Build history of the part. All positions in model axes, mm. A direction names the side the tool comes from. Round coordinates to 2 decimals unless told otherwise and drop trailing zeros. Write each loop counter-clockwise with the first axis right and the second up, starting at its lowest first coordinate (ties: lowest second). Pieces come first, ordered by that corner, then holes. Notation, with made-up numbers: M 61,2 L 69,2 A23 ccw 69,24 Z; hole C 17.25,83.5 d9. An arc over 180 degrees is marked long. Write item = value, one per line.
from build123d import *

# Parameters (mm, degrees)
SKETCH1_W           = 304.8
SKETCH1_H           = 381
BOSS_EXTRUDE1_DEPTH = 152.4
SKETCH2_R           = 38.1
CUT_EXTRUDE1_DEPTH  = 50.8
SKETCH5_W           = 152.4
SKETCH5_H           = 101.6
BOSS_EXTRUDE3_DEPTH = 127
SKETCH6_R           = 25.4
CUT_EXTRUDE4_DEPTH  = 50.8
FILLET4_R           = 25.4
FILLET5_R           = 25.4
SKETCH3_R           = 38.1
BOSS_EXTRUDE4_DEPTH = 44.45
SKETCH8_W           = 122.871403684
SKETCH8_H           = 31.75
CUT_EXTRUDE5_DEPTH  = 63.5
SKETCH9_R           = 12.7
BOSS_EXTRUDE5_DEPTH = 32.766


with BuildPart() as part:
    # Sketch1 → Boss-Extrude1 (new body)
    with BuildSketch(Plane.XY):
        Rectangle(SKETCH1_W, SKETCH1_H)
    extrude(amount=BOSS_EXTRUDE1_DEPTH)

    # Sketch2 → Cut-Extrude1 (cut)
    with BuildSketch(Plane(origin=(0, 190.5, 0), x_dir=(1, 0, 0), z_dir=(0, 1, 0))):
        with Locations(Location((0, -76.2, 0), (0, 0, 270))):
            Circle(SKETCH2_R)
    extrude(amount=-CUT_EXTRUDE1_DEPTH, mode=Mode.SUBTRACT)

    # Sketch5 → Boss-Extrude3 (add)
    with BuildSketch(Plane(origin=(152.4, 0, 0), x_dir=(0, 0, -1), z_dir=(1, 0, 0))):
        with Locations((-76.2, 139.7)):
            Rectangle(SKETCH5_W, SKETCH5_H)
    boss_extrude3 = extrude(amount=BOSS_EXTRUDE3_DEPTH)

    # Mirror1: Boss-Extrude3 across plane
    add(boss_extrude3.mirror(Plane(origin=(0, 0, 0), x_dir=(0, 0, 1), z_dir=(1, 0, 0))))

    # Sketch6 → Cut-Extrude4 (cut)
    with BuildSketch(Plane.XZ.offset(-88.9)):
        with Locations(Location((228.6, 76.2, 0), (0, 0, 270))):
            Circle(SKETCH6_R)
    cut_extrude4 = extrude(amount=-CUT_EXTRUDE4_DEPTH, mode=Mode.SUBTRACT)

    # Fillet4
    fillet4_edges = [part.edges().sort_by_distance(p)[0] for p in [
        (279.4, 190.5, 76.2),
        (-279.4, 190.5, 76.2),
    ]]
    fillet(fillet4_edges, radius=FILLET4_R)

    # Fillet5
    fillet5_edges = [part.edges().sort_by_distance(p)[0] for p in [
        (-152.4, -190.5, 76.2),
        (152.4, -190.5, 76.2),
    ]]
    fillet(fillet5_edges, radius=FILLET5_R)

    # Mirror2: Cut-Extrude4 across plane
    add(cut_extrude4.mirror(Plane(origin=(0, 0, 0), x_dir=(0, 0, 1), z_dir=(1, 0, 0))), mode=Mode.SUBTRACT)

    # Sketch3 → Boss-Extrude4 (add)
    with BuildSketch(Plane.XZ.offset(190.5)):
        with Locations(Location((-101.6, 76.2, 0), (0, 0, 131.810314896))):
            Circle(SKETCH3_R)
        with Locations(Location((101.6, 76.2, 0), (0, 0, 48.189685104))):
            Circle(SKETCH3_R)
    extrude(amount=BOSS_EXTRUDE4_DEPTH)

    # Sketch8 → Cut-Extrude5 (cut)
    with BuildSketch(Plane.XZ.offset(234.95)):
        with Locations((101.6, 76.2)):
            Rectangle(SKETCH8_W, SKETCH8_H)
    cut_extrude5 = extrude(amount=-CUT_EXTRUDE5_DEPTH, mode=Mode.SUBTRACT)

    # Mirror3: Cut-Extrude5 across plane
    add(cut_extrude5.mirror(Plane(origin=(0, 0, 0), x_dir=(0, 0, 1), z_dir=(1, 0, 0))), mode=Mode.SUBTRACT)

    # Sketch9 → Boss-Extrude5 (add)
    with BuildSketch(Plane.XY.offset(60.325)):
        with Locations(Location((102.203286199, -221.696968448, 0), (0, 0, 180))):
            Circle(SKETCH9_R)
    boss_extrude5 = extrude(amount=BOSS_EXTRUDE5_DEPTH)

    # Mirror4: Boss-Extrude5 across plane
    add(boss_extrude5.mirror(Plane(origin=(0, 0, 0), x_dir=(0, 0, 1), z_dir=(1, 0, 0))))


solid = part.part
1. Band-saw the part on B-B (z = 69). Count the separate pieces of the cut face and the enclosed holes in it, plus the area to 3 significant figures.
Responses:
separate_pieces = 3
enclosed_holes = 0
area = 130,000 mm²
2. Flat gauge pins, fed straight in: pin 1 (5.5 mm diameter, centred on y = -176.5, z = 83.5, fed in from +X); pin 2 (4 mm diameter, centred on y = 20, z = 78, fed in from -X); pin 3 (16 mm diameter, centred on x = -121, z = 76, fed in from -Y). Where does each tip first touch, or does it go through?
Responses:
pin_1 = 40.16
pin_2 = -152.4
pin_3 = -228.38
3. Tool access for faces 4 (the face through (102.209, -212.414, 114.295)), 5 (the face through (-95, -197, 92.075)), 6 (the face through (-152.4, -40, 75)), 7 (the face through (229, 139.7, 77)): list every direction of +Z, -Z, +X, -X, +Y, -Y with a clear straight run to the whole face (end or side of a thin tool).
Responses:
face_4 = +Z, -Y
face_5 = none
face_6 = +Z, -Z, -X, -Y
face_7 = -Y
4. Mould opens along Z. For faces 1 (the face through (271.76, 183.26, 75.13)), 2 (the face through (100.991, -212.414, 38.105)), 3 (the face through (95, -171.45, 76)) say: pulls with the +Z half, pulls with the -Z half, needs draft (parallel to the pull), parting line crosses it, or undercut.
Responses:
face_1 = needs draft
face_2 = pulls with the -Z half
face_3 = undercut
5. Band-saw the part on D-D (y = -56.5). List the corners of the cut face in (x, z).
Responses:
outline = M -152.4,0 L 152.4,0 L 152.4,152.4 L -152.4,152.4 Z
6. Band-saw the part on A-A (z = 15). List the corners of the cut face in (x, y).
Responses:
outline = M -279.4,88.9 L -152.4,88.9 L -152.4,-165.1 A25.4 ccw -127,-190.5 L 127,-190.5 A25.4 ccw 152.4,-165.1 L 152.4,88.9 L 279.4,88.9 L 279.4,165.1 A25.4 ccw 254,190.5 L -254,190.5 A25.4 ccw -279.4,165.1 Z
7. Band-saw the part on C-C (x = 0). List the corners of the cut face in (y, z), plus the area to 3 significant figures.
Responses:
outline = M -190.5,0 L 190.5,0 L 190.5,38.1 L 139.7,38.1 L 139.7,114.3 L 190.5,114.3 L 190.5,152.4 L -190.5,152.4 Z
area = 54,200 mm²
8. Probe probe 1 along X at (y, z) = (117, 76.2); probe 2 along Z at (x, y) = (-58, -174) (3 decimals); probe 3 along X at (y, z) = (160.5, 76.2). List the from-to ranges inside material, lowest first.
Responses:
probe_1 = -279.4 to -254, -203.2 to 203.2, 254 to 279.4
probe_2 = 0 to 60.325, 92.075 to 152.4
probe_3 = -279.4 to -38.1, 38.1 to 279.4
